Design review of the part shown in the three views and the two pictorial views. Dimensions are in mm from the part's minimum x, y and z. A direction names the side the tool comes from. Coordinates: 2 decimals unless noted, no trailing zeros. Loops run counter-clockwise (first coordinate to the right, second up) from the corner with the lowest first, then second, coordinate; pieces in that order, holes last. Notation, with made-up numbers: (-38.75, -31) -> (-28.75, -31) arc R8 ccw to (-28.75, -26) -> close; hole circle Ø5 at (3.25, -27). An arc over 180 degrees is marked (long way). Use CSV: the item, a comma, the result in double quotes.
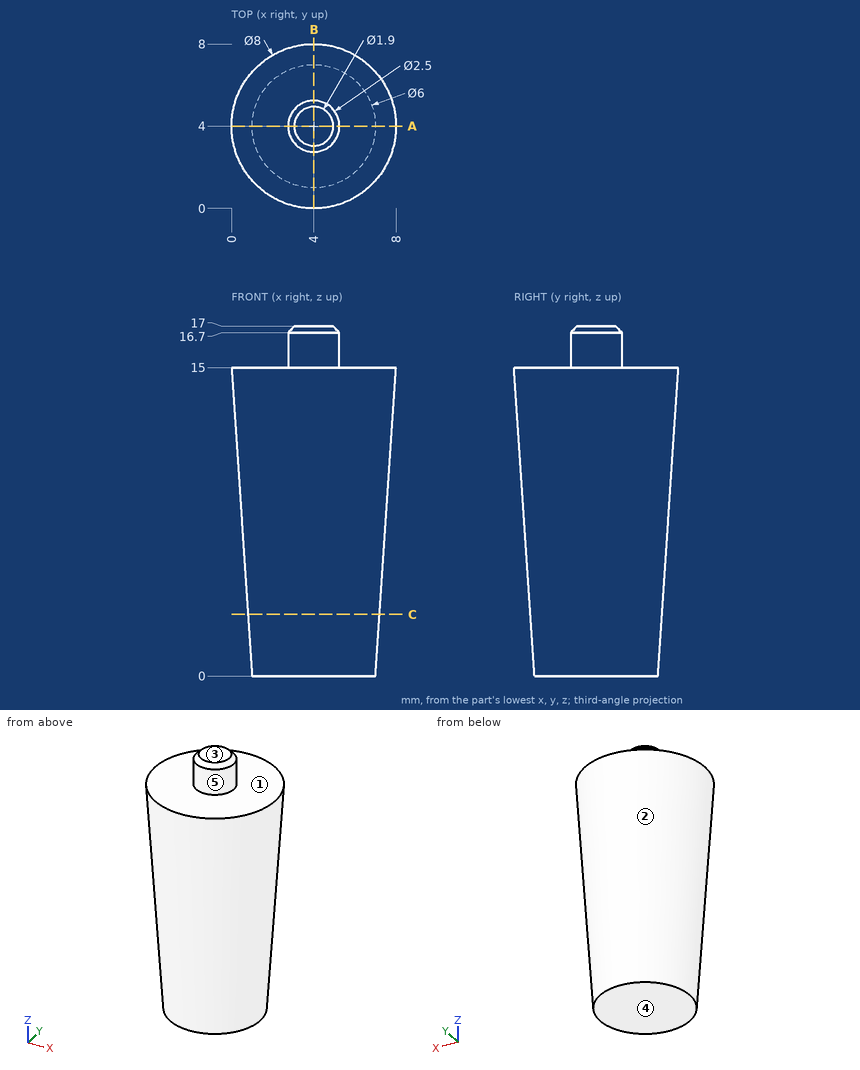
Item 1: Add section A-A (y = 4). Give the boundary of the cut face in (x, z), then the cut area to 3 significant figures.
Checked values:
outline,"(0, 15) -> (1, 0) -> (7, 0) -> (8, 15) -> (5.25, 15) -> (5.25, 16.7) -> (4.95, 17) -> (3.05, 17) -> (2.75, 16.7) -> (2.75, 15) -> close"
area,"110 mm^2"
Item 2: To check wall thickness, follow line 1 along Z through (x, y) = (2.75, 5.5); line 2 along X through (y, z) = (4.5, 11); line 3 along Y through (x, z) = (7, 7.25). State the ranges of each line that lie inside material, in increasing order.
Checked values:
line 1,"0 to 15"
line 2,"0.3 to 7.7"
line 3,"2.23 to 5.77"
Item 3: Machinability: for the marked faces 1 and 2, which of the approach directions +Z, -Z, +X, -X, +Y, -Y give a long, thin tool a straight path to every point of the face, cutting with its end or side? Answer none if there is none.
Checked values:
face 1,"+Z"
face 2,"-Z"
Item 4: Clearance check with flat-ended pins moving along their axes: pin 1 (1.5 mm diameter, centred on x = 5, z = 13, fed in from +Y); pin 2 (2 mm diameter, centred on x = 3.5, y = 6, fed in from +Z); pin 3 (1.5 mm diameter, centred on y = 7, z = 15, fed in from +X). State where each tip first meets the part, or that it passes through.
Checked values:
pin 1,"y = 7.88"
pin 2,"z = 16.89"
pin 3,"x = 7.31"
Item 5: Add section C-C (z = 3). Give the boundary of the cut face in (x, y).
Checked values:
outline,"circle Ø6.4 at (4, 4)"
Item 6: Draft analysis for pull direction Z (two halves, no side actions). For the marked faces 3, 4 and 5, state which applies: pulls with the +Z half, pulls with the -Z half, needs draft (parallel to the pull), parting line crosses it, or undercut.
Checked values:
face 3,"pulls with the +Z half"
face 4,"pulls with the -Z half"
face 5,"needs draft"
